from build123d import *

# Parameters (mm, degrees)
SKETCH_4_OUTSIDE_W  = 67.78
SKETCH_4_OUTSIDE_H  = 67.78
CUT_EXTRUDE_1_DEPTH = 7


with BuildPart() as part:
    # Эскиз1 → Повернуть1 (revolve)
    with BuildSketch(Plane.XY, mode=Mode.PRIVATE) as revolve_1_sk:
        with BuildLine():
            Line((0, 21.68), (0, 25))
            Line((0, 25), (-27, 25))
            Line((-27, 25), (-27, 21))
            Line((-27, 21), (-35, 21))
            Line((-35, 21), (-35, 2))
            Line((-35, 2), (-24, 2))
            Line((-24, 2), (-24, 14))
            Line((-24, 14), (-20, 14))
            Line((-20, 14), (-20, 20.45))
            ThreePointArc((-20, 20.45), (-19.765685425, 21.015685425), (-19.2, 21.25))
            Line((-19.2, 21.25), (-14.33137085, 21.25))
            ThreePointArc((-14.33137085, 21.25), (-14.025224104, 21.189103626), (-13.765685425, 21.015685425))
            Line((-13.765685425, 21.015685425), (-12.83, 20.08))
            Line((-12.83, 20.08), (-1.6, 20.08))
            Line((-1.6, 20.08), (0, 21.68))
        make_face()
    revolve(revolve_1_sk.sketch.rotate(Axis((0, 0, 0), (-1, 0, 0)), 90), axis=Axis((0, 0, 0), (-1, 0, 0)))

    # Эскиз4 outside → Вырез-Вытянуть1 (cut)
    with BuildSketch(Plane.ZY.offset(35)):
        Rectangle(SKETCH_4_OUTSIDE_W, SKETCH_4_OUTSIDE_H)
        Polygon((20.784609691, 0), (10.392304845, 18), (-10.392304845, 18), (-20.784609691, 0), (-10.392304845, -18), (10.392304845, -18), align=None, mode=Mode.SUBTRACT)
    extrude(amount=-CUT_EXTRUDE_1_DEPTH, mode=Mode.SUBTRACT)


solid = part.part
Build history of the part. All positions in model axes, mm. A direction names the side the tool comes from. Round coordinates to 2 decimals unless told otherwise and drop trailing zeros. Write each loop counter-clockwise with the first axis right and the second up, starting at its lowest first coordinate (ties: lowest second). Pieces come first, ordered by that corner, then holes. Notation, with made-up numbers: (-20.75, 59) -> (22.25, 59) arc R14 cw to (22.25, 77) -> close; hole circle Ø8 at (14, 54). An arc over 180 degrees is marked (long way). Write item = value, one per line.
(1) Two-plate mould, pull along Z, no slides. Class faces 1 (the face through (-16.73, -6.38, -20.27)), 2 (the face through (-27.51, -6.31, -20.03)), 3 (the face through (-7.14, -0.88, 20.06)), 4 (the face through (-35, 0, -4)): pulls with the +Z half, pulls with the -Z half, needs draft (parallel to the pull), parting line crosses it, or undercut.
Answer:
face_1 = undercut
face_2 = parting line crosses it
face_3 = undercut
face_4 = needs draft
(2) Band-saw the part on C-C (x = -15.5). Give the cut face in (y, z), then the cut area to 3 significant figures.
Answer:
outline = circle Ø50 at (0, 0); hole circle Ø42.5 at (0, 0)
area = 545 mm2
(3) Probe L1, parallel to Y at x = -9.25, z = 0; L2, parallel to Y at x = -21.65, z = 0; L3, parallel to X at y = 10.5, z = 18. List the from-to ranges inside material, lowest first.
Answer:
L1 = -25 to -20.08, 20.08 to 25
L2 = -25 to -14, 14 to 25
L3 = -28 to -19.9, -13.59 to -0.84
(4) Flat gauge pins, fed straight in: pin 1 (6 mm diameter, centred on x = -11.5, z = 8, fed in from -Y); pin 2 (1.5 mm diameter, centred on x = -24.5, y = 18.5, fed in from -Z); pin 3 (6 mm diameter, centred on x = -18, z = 17, fed in from +Y); pin 4 (3.5 mm diameter, centred on y = 0, z = 0, fed in from -X). Where does each tip first touch, or does it go through?
Answer:
pin_1 = -24.49
pin_2 = -17.61
pin_3 = 20.71
pin_4 = through
(5) Tool access for faces 5 (the face through (-31.549, 9.126, -15.516)), 6 (the face through (-31.549, -9.126, 15.516)), 7 (the face through (-22, 12.4, -6.5)), 8 (the face through (-27, -20.5, 5.7)): list every direction of +Z, -Z, +X, -X, +Y, -Y with a clear straight run to the whole face (end or side of a thin tool).
Answer:
face_5 = -Z, -X, +Y
face_6 = +Z, -X, -Y
face_7 = +X
face_8 = -X
(6) Band-saw the part on D-D (x = -23). Give the cut face in (y, z).
Answer:
outline = circle Ø50 at (0, 0); hole circle Ø28 at (0, 0)
(7) Band-saw the part on B-B (x = -30). Give the cut face in (y, z).
Answer:
outline = (-18, -10.39) -> (0, -20.78) -> (18, -10.39) -> (18, 10.39) -> (0, 20.78) -> (-18, 10.39) -> close; hole circle Ø4 at (0, 0)
